from build123d import *

# Parameters (mm, degrees)
ESQUISSE1_R                  = 10
BOSS_EXTRU_1_DEPTH           = 40
ESQUISSE2_R                  = 0.75
ENL_V_MAT_EXTRU_1_DEPTH      = 40
ENL_V_MAT_EXTRU_1_DEPTH_BACK = 40
ESQUISSE3_R                  = 5.241374435
BOSS_EXTRU_2_DEPTH           = 20
ESQUISSE4_R                  = 3.5
BOSS_EXTRU_3_DEPTH           = 9
ESQUISSE5_R                  = 4.3
BOSS_EXTRU_4_DEPTH           = 4
CONG_2_R                     = 2


with BuildPart() as part:
    # Esquisse1 → Boss.-Extru.1 (new body)
    with BuildSketch(Plane.XY):
        Circle(ESQUISSE1_R)
        Polygon((4.156921938, 0), (2.078460969, 3.6), (-2.078460969, 3.6), (-4.156921938, 0), (-2.078460969, -3.6), (2.078460969, -3.6), align=None, mode=Mode.SUBTRACT)
    extrude(amount=BOSS_EXTRU_1_DEPTH)

    # Esquisse2 → Enlèv. mat.-Extru.1 (cut, two sides)
    with BuildSketch(Plane(origin=(0, 0, 0), x_dir=(1, 0, 0), z_dir=(0, 1, 0))) as enl_v_mat_extru_1_sk:
        with Locations((0, -8)):
            Circle(ESQUISSE2_R)
    extrude(amount=ENL_V_MAT_EXTRU_1_DEPTH, mode=Mode.SUBTRACT)
    extrude(enl_v_mat_extru_1_sk.sketch, amount=-ENL_V_MAT_EXTRU_1_DEPTH_BACK, mode=Mode.SUBTRACT)

    # Esquisse3 → Boss.-Extru.2 (add)
    with BuildSketch(Plane.XY.offset(40)):
        Circle(ESQUISSE3_R)
    extrude(amount=-BOSS_EXTRU_2_DEPTH)

    # Esquisse4 → Boss.-Extru.3 (add)
    with BuildSketch(Plane.XY.offset(40)):
        Circle(ESQUISSE4_R)
    extrude(amount=BOSS_EXTRU_3_DEPTH)

    # Esquisse5 → Boss.-Extru.4 (add)
    with BuildSketch(Plane.XY.offset(40)):
        Circle(ESQUISSE5_R)
    extrude(amount=BOSS_EXTRU_4_DEPTH)

    # Congé2
    cong_2_edges = [part.edges().sort_by_distance(p)[0] for p in [
        (-4.3, 0, 40),
    ]]
    fillet(cong_2_edges, radius=CONG_2_R)


solid = part.part
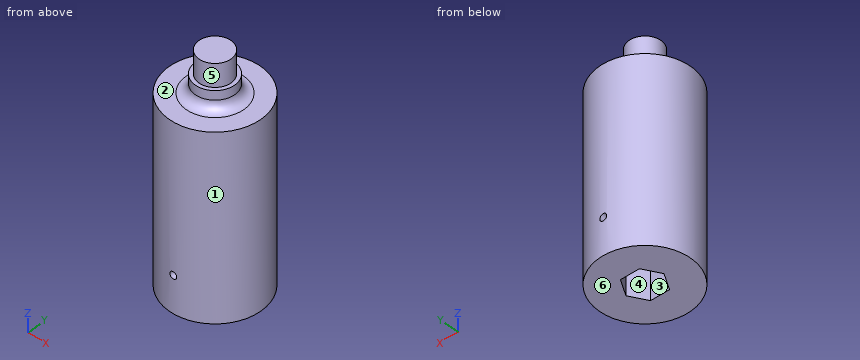
Build history of the part. All positions in model axes, mm. Face numbers are marked on the shaded views. A direction names the side the tool comes from. Round coordinates to 2 decimals unless told otherwise and drop trailing zeros. Loops run counter-clockwise (first coordinate to the right, second up) from the corner with the lowest first, then second, coordinate; pieces in that order, holes last. Notation, with made-up numbers: (-1, 60.25) -> (39, 60.25) arc R20 cw to (39, 96.25) -> close; hole circle Ø6 at (8.25, -27.75). An arc over 180 degrees is marked (long way). One line per item, written item: value. Start each with the question number.
Q1. Cut at C-C on z = 39.5. List the corners of the cut face in (x, y), plus the area to 3 significant figures.
Q2. Probe line 1 along Z through (x, y) = (0, 6.5); line 2 along Z through (x, y) = (-7.5, -1.25); line 3 along X through (y, z) = (-8, 8). List the from-to ranges inside material, lowest first.
Q3. Cut at B-B on z = 8. List the corners of the cut face in (x, y), plus the area to 3 significant figures.
Q4. 3-axis set-ups, long thin cutter, end or side, ignore diameter. For the marked faces 1, 2 and 3: which of +Z, -Z, +X, -X, +Y, -Y reach the whole face in a straight line?
Q5. Cut at A-A on x = 0. List the corners of the cut face in (y, z), plus the area to 3 significant figures.
Q6. Two-plate mould, pull along Y, no slides. Class the marked faces 4, 5 and 6: released by +Y, released by -Y, zero draft, split by the parting line, or undercut.
Q7. Drop flat-ended pins along their axis: pin 1 Ø6 at (x, z) = (-4.5, 12.5) entering from -Y; pin 2 Ø1 at (x, z) = (-5, 33) entering from +Y; pin 3 Ø6 at (x, y) = (-0.5, 0) entering from -Z. Give the stop position or say it passes through.
Computed:
1. outline: circle Ø20 at (0, 0)
1. area: 314 mm²
2. line 1: 0 to 7.25, 8.75 to 40
2. line 2: 0 to 40
2. line 3: -6 to -0.75, 0.75 to 6
3. outline: (-4.16, 0) -> (-2.08, 3.6) -> (-0.75, 3.6) -> (-0.75, 9.97) arc R10 ccw to (-0.75, -9.97) -> (-0.75, -3.6) -> (-2.08, -3.6) -> close; (0.75, -9.97) arc R10 ccw to (0.75, 9.97) -> (0.75, 3.6) -> (2.08, 3.6) -> (4.16, 0) -> (2.08, -3.6) -> (0.75, -3.6) -> close
3. area: 250 mm²
4. face 1: +Z, -Z
4. face 2: +Z
4. face 3: -Z
5. outline: (-10, 0) -> (-3.6, 0) -> (-3.6, 7.25) -> (-10, 7.25) -> close; (-10, 8.75) -> (-3.6, 8.75) -> (-3.6, 20) -> (3.6, 20) -> (3.6, 8.75) -> (10, 8.75) -> (10, 40) -> (6.3, 40) arc R2 cw to (4.3, 42) -> (4.3, 44) -> (3.5, 44) -> (3.5, 49) -> (-3.5, 49) -> (-3.5, 44) -> (-4.3, 44) -> (-4.3, 42) arc R2 cw to (-6.3, 40) -> (-10, 40) -> close; (3.6, 0) -> (10, 0) -> (10, 7.25) -> (3.6, 7.25) -> close
5. area: 708 mm²
6. face 4: undercut
6. face 5: split by the parting line
6. face 6: zero draft
7. pin 1: y = -9.89
7. pin 2: y = 8.93
7. pin 3: z = 20
